For this review, take the finished solid that the model builds, in its own axes (mm). A direction names the side the tool comes from. Give positions to 0.01 mm unless a question says otherwise; leave off trailing zeros. Order: outer loops, then holes, each group sorted by start corner. A loop starts at its lowest first (then second) coordinate and runs counter-clockwise, first axis right, second up. Notation, with made-up numbers: M 88,34.25 L 98,34.25 A32 ccw 98,72.25 Z; hole C 8.5,36.5 d4. An arc over 180 degrees is marked long. Use CSV: the item, a comma, the result in double quotes. Start each with the question number.
(1) Clearance check with flat-ended pins moving along their axes: P1, Ø12, axis at y = 286.5, z = 22, coming from the +X side; P2, Ø4, axis at x = 25, z = 29, coming from the +Y side; P3, Ø11.5, axis at x = 26, y = 299, coming from the -Z side; P4, Ø7.5, axis at x = 20.5, z = 9.5, coming from the -Y side. State where each tip first meets the part, or that it passes through.
(2) Wall thickness on L1, parallel to Z at x = 33, y = 257; L2, parallel to Y at x = 13, z = 73; L3, parallel to Y at x = 23, z = 65.5: over which ranges is each line inside the solid? List them lowest first. Write a range as from..to.
(3) Consider section B-B (z = 13.5). Write out the cut boundary in (x, y), and give its area (3 significant figures).
(4) Consider section A-A (x = 31). Write out the cut boundary in (y, z), and give its area (3 significant figures).
(5) Draft analysis for pull direction Y (two halves, no side actions). For faces 1 (the face through (19, 19, 44)), 2 (the face through (19, 152.4, 13)), 3 (the face through (0, 258, 44)), state which applies: pulls with the +Y half, pulls with the -Y half, needs draft (parallel to the pull), parting line crosses it, or undercut.
(6) Consider section D-D (x = 11.5). Write out the cut boundary in (y, z), and give its area (3 significant figures).
(7) Consider section C-C (y = 269). Write out the cut boundary in (x, z), and give its area (3 significant figures).
(8) Tool access review of faces 4 (the face through (19, 253, 25.4)), 5 (the face through (19, 489, 44)): name each direction out of +Z, -Z, +X, -X, +Y, -Y from which nothing blocks a thin tool from reaching the whole face with its end or side.
```python
from build123d import *

# Parameters (mm, degrees)
F1_DEPTH = 88.9
F2_W     = 203.2
F2_H     = 50.8
F3_DEPTH = 72.804831


with BuildPart() as f1:
    # F0 (on Top) → F1 (new body)
    with BuildSketch(Plane.XY):
        Polygon((0, 508), (0, 0), (38.1, 38.1), (38.1, 469.9), align=None)
    extrude(amount=F1_DEPTH)

    # F2 (on face) → F3 (cut)
    with BuildSketch(Plane.YZ.offset(38.1)):
        with Locations((254, 0)):
            Rectangle(F2_W, F2_H)
    extrude(amount=-F3_DEPTH, mode=Mode.SUBTRACT)


solid = f1.part
```
Check result:
1,P1,"stops at x = 38.1"
1,P2,"stops at y = 485"
1,P3,"stops at z = 25.4"
1,P4,"stops at y = 16.75"
2,L1,"z = 25.4..88.9"
2,L2,"y = 13..495"
2,L3,"y = 23..485"
3,outline,"M 0,0 L 38.1,38.1 L 38.1,152.4 L 0,152.4 Z; M 0,355.6 L 38.1,355.6 L 38.1,469.9 L 0,508 Z"
3,area,"10,200 mm^2"
4,outline,"M 31,0 L 152.4,0 L 152.4,25.4 L 355.6,25.4 L 355.6,0 L 477,0 L 477,88.9 L 31,88.9 Z"
4,area,"34,500 mm^2"
5,face 1,"pulls with the -Y half"
5,face 2,"undercut"
5,face 3,"needs draft"
6,outline,"M 11.5,0 L 152.4,0 L 152.4,25.4 L 355.6,25.4 L 355.6,0 L 496.5,0 L 496.5,88.9 L 11.5,88.9 Z"
6,area,"38,000 mm^2"
7,outline,"M 0,25.4 L 38.1,25.4 L 38.1,88.9 L 0,88.9 Z"
7,area,"2,420 mm^2"
8,face 4,"-Z, +X, -X"
8,face 5,"+Z, -Z, +X, +Y"
